Part model, mm, in its own coordinate system. Face numbers are marked on the shaded views. Give positions to 0.01 mm unless a question says otherwise; leave off trailing zeros. Order: outer loops, then holes, each group sorted by start corner. A loop starts at its lowest first (then second) coordinate and runs counter-clockwise, first axis right, second up. Notation, with made-up numbers: (66.25, 49.5) -> (88.25, 49.5) arc R15 ccw to (88.25, 62.5) -> close; hole circle Ø6 at (12, 77.5). An arc over 180 degrees is marked (long way). Write item = value, one per line. Start each with the question number.
Item 1: Flat gauge pins, fed straight in: P1, Ø3.5, axis at x = -1.5, z = 0, coming from the +Y side; P2, Ø1, axis at x = 1.5, y = 2, coming from the +Z side; P3, Ø2, axis at x = -0.5, y = 2.5, coming from the +Z side; P4, Ø1, axis at x = 2, y = 1.5, coming from the +Z side. Where does each tip first touch, or does it go through?
Item 2: Band-saw the part on A-A on y = 3.3. Write the cut outline in (x, z).
Item 3: Drill centre lines: line 1 along X through (y, z) = (2.25, 0); line 2 along Y through (x, z) = (-1.5, 2.5); line 3 along X through (y, z) = (1.3, 0.5). Where is each one in solid material? Low to high.
Item 4: Band-saw the part on C-C on z = 3. Write the cut outline in (x, y), plus the area to 3 significant figures.
Item 5: Band-saw the part on B-B on y = 3.8. Write the cut outline in (x, z), plus the area to 3 significant figures.
Item 6: Pull direction Z, two halves, no side cores. Call the marked faces 1, 2 and 3: +Z half, -Z half, draft (parallel to the pull), parting line (faces both ways), or undercut.
```python
from build123d import *

# Parameters (mm, degrees)
DOME_2_FACE_RADIUS = 2.75
DOME_2_HEIGHT      = 0.5
FILLET_1_R         = 0.3


with BuildPart() as part:
    # 草图1 → 旋转2 (revolve)
    with BuildSketch(Plane.XY, mode=Mode.PRIVATE) as revolve_2_sk:
        Polygon((-3.7, 0), (-1.6, 0), (-1.6, 3.5), (0, 3.5), (0, 4.5), (-2.75, 4.5), (-2.75, 0.5), (-3.7, 0.5), align=None)
    revolve(revolve_2_sk.sketch.rotate(Axis((0, -1.216580074, 0), (0, 1, 0)), 270), axis=Axis((0, -1.216580074, 0), (0, 1, 0)))

    # 圆顶2: a dome of height H over a round flat face of radius A is a cap of a sphere of radius (A * A + H * H) / (2 * H)
    dome_2_r = (DOME_2_FACE_RADIUS * DOME_2_FACE_RADIUS + DOME_2_HEIGHT * DOME_2_HEIGHT) / (2 * DOME_2_HEIGHT)
    dome_2_base = Plane((0, 4.5, 0), z_dir=(0, 1, 0))
    with Locations(dome_2_base.offset(DOME_2_HEIGHT - dome_2_r)):
        dome_2_ball = Sphere(dome_2_r, mode=Mode.PRIVATE)
    add(split(dome_2_ball, bisect_by=dome_2_base, keep=Keep.TOP, mode=Mode.PRIVATE))

    # 圆角1
    fillet_1_edges = [part.edges().sort_by_distance(p)[0] for p in [
        (2.75, 4.5, 0),
    ]]
    fillet(fillet_1_edges, radius=FILLET_1_R)


solid = part.part
```
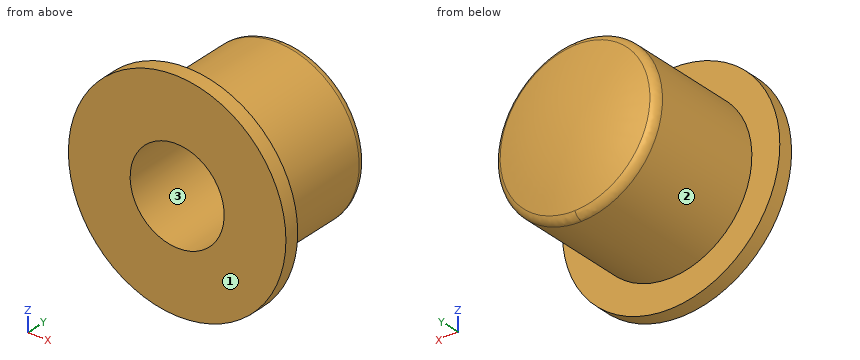
Values found:
q1.P1 = 5
q1.P2 = 2.56
q1.P3 = 2.75
q1.P4 = 2.3
q2.outline = circle Ø5.5 at (0, 0); hole circle Ø3.2 at (0, 0)
q3.line_1 = -2.75 to -1.6, 1.6 to 2.75
q3.line_2 = 0 to 0.5
q3.line_3 = -2.7 to -1.52, 1.52 to 2.7
q4.outline = (-2.17, 0) -> (2.17, 0) -> (2.17, 0.5) -> (-2.17, 0.5) -> close
q4.area = 2.17 mm^2
q5.outline = circle Ø5.5 at (0, 0)
q5.area = 23.8 mm^2
q6.face_1 = draft
q6.face_2 = parting line
q6.face_3 = undercut
